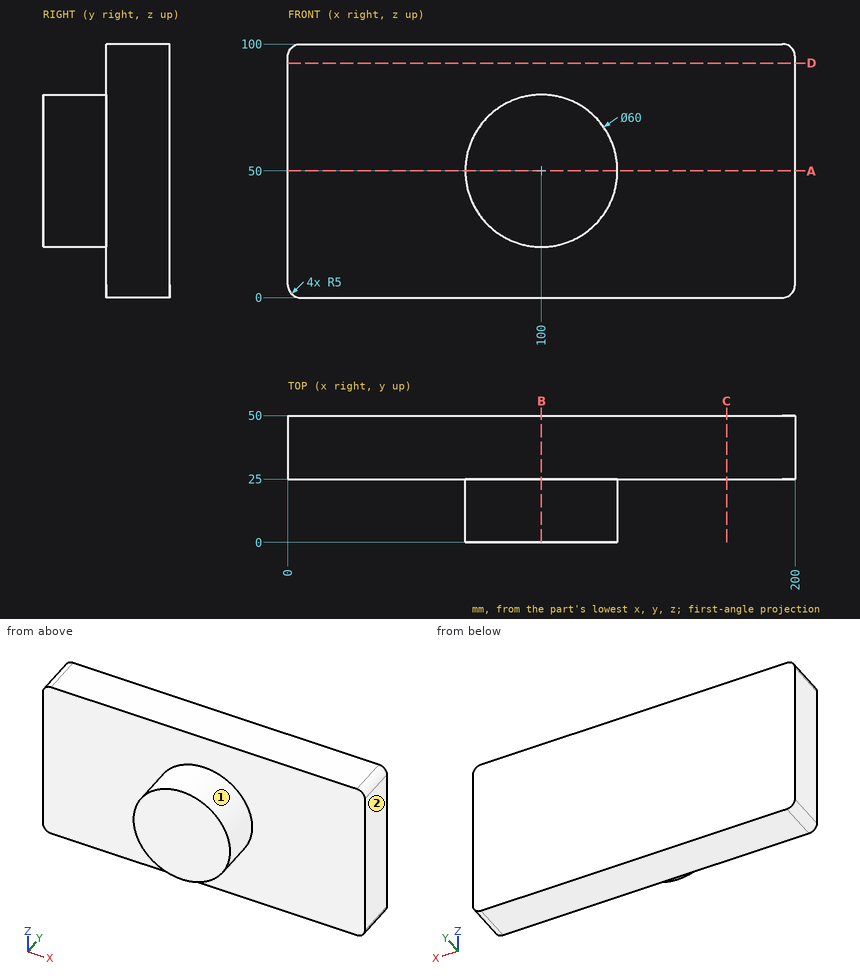
Answer from the drawing. Dimensions are ordinates in mm from the lowest x, y and z of the part. A direction names the side the tool comes from. Coordinates: 2 decimals unless noted, no trailing zeros. Order: outer loops, then holes, each group sorted by start corner. A loop starts at its lowest first (then second) coordinate and runs counter-clockwise, first axis right, second up. Notation, with made-up numbers: (-7, 70.5) - (12, 70.5) arc R25 ccw to (12, 104.5) - close; hole circle Ø5 at (-3.5, 2.5). An arc over 180 degrees is marked (long way). Answer as a JSON object with one key per item and string values. Group by question number.
Item 1: Section C-C (x = 173) is taken. Give the vertices of the cut face in (y, z), plus the area to 3 significant figures.
Item 2: A flat-ended cylindrical pin translates along its axis: P1, Ø1, axis at x = 26, z = 24, coming from the -Y side. Find the tip coordinate at first contact, or state that the pin passes through.
Item 3: Section A-A (z = 50) is taken. Give the vertices of the cut face in (x, y), plus the area to 3 significant figures.
Item 4: A tool of negligible diameter and unlimited length cuts with its end or side. For the marked faces 1 and 2, from which of +Z, -Z, +X, -X, +Y, -Y can it reach the whole face along a straight path? Write none if from no direction.
Item 5: Section D-D (z = 92.5) is taken. Give the vertices of the cut face in (x, y).
Item 6: Consider probe 1 along Y at (x, z) = (108.5, 80.5); probe 2 along Z at (x, y) = (126.5, 5); probe 3 along X at (y, z) = (17, 30.5). Determine where each line is inside the solid, lowest interval first. Write a range as from..to.
Item 7: Section B-B (x = 100) is taken. Give the vertices of the cut face in (y, z).
Results are:
{
 "1": {"outline": "(25, 0) - (50, 0) - (50, 100) - (25, 100) - close", "area": "2,500 mm^2"},
 "2": {"P1": "stops at y = 25"},
 "3": {"outline": "(0, 25) - (70, 25) - (70, 0) - (130, 0) - (130, 25) - (200, 25) - (200, 50) - (0, 50) - close", "area": "6,500 mm^2"},
 "4": {"face 1": "-Y", "face 2": "+Z, -Z, +X, +Y, -Y"},
 "5": {"outline": "(0, 25) - (200, 25) - (200, 50) - (0, 50) - close"},
 "6": {"probe 1": "y = 25..50", "probe 2": "z = 35.94..64.06", "probe 3": "x = 77.2..122.8"},
 "7": {"outline": "(0, 20) - (25, 20) - (25, 0) - (50, 0) - (50, 100) - (25, 100) - (25, 80) - (0, 80) - close"}
}
